Geometry check sheet. Reference: the model listing, model coordinates, mm. Face numbers are marked on the shaded views. A direction names the side the tool comes from. Give positions to 0.01 mm unless a question says otherwise; leave off trailing zeros. Loops run counter-clockwise (first coordinate to the right, second up) from the corner with the lowest first, then second, coordinate; pieces in that order, holes last.
1. Cross-section at C-C, the plane z = 0.8. Record the cut outline in (x, y).
2. Go/stop test with a flat-tipped pin: pin 1 Ø1 at (x, y) = (2.5, 5) entering from +Z. Record where the tip stops, or that it passes through.
3. Material ranges on L1, parallel to Y at x = -1.75, z = 1.2; L2, parallel to Y at x = -4, z = 4.7; L3, parallel to X at y = 0.5, z = 3.1, recorded low to high.
4. Cross-section at A-A, the plane y = 0.25. Record the cut outline in (x, z).
5. Cross-section at B-B, the plane x = -4. Record the cut outline in (y, z).
6. Cross-section at D-D, the plane x = 0.25. Record the cut outline in (y, z), plus the area to 3 significant figures.
7. Tool access check on the marked faces 1, 2 and 3. Record the directions out of +Z, -Z, +X, -X, +Y, -Y that give a thin tool (end or side, any length) a straight path to the whole face; none if there is none.
8. Release check for a two-part mould opening along Y. For the marked faces 4, 5, 6 and 7 record: +Y half, -Y half, draft (parallel to the pull), parting line (faces both ways), or undercut.
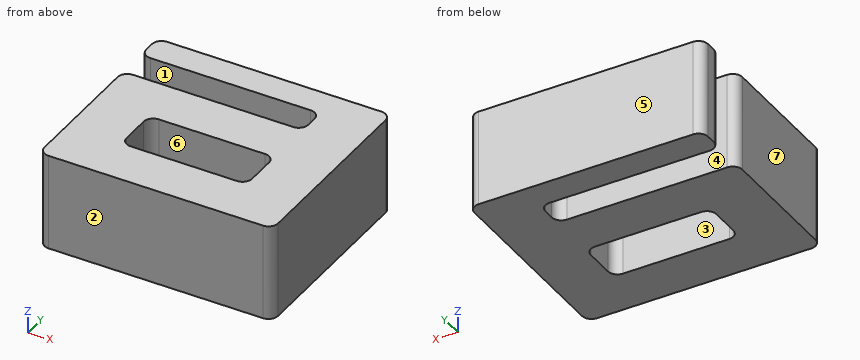
from build123d import *

# Parameters (mm, degrees)
SKETCH1_W           = 6.5
SKETCH1_H           = 2.5
BOSS_EXTRUDE1_DEPTH = 5
FILLET1_R           = 0.5


with BuildPart() as part:
    # Sketch1 → Boss-Extrude1 (new body)
    with BuildSketch(Plane.XY):
        Polygon((-6.05, -3.75), (6.05, -3.75), (6.05, 6.8), (-6.05, 6.8), (-6.05, 5.3), (3.25, 5.3), (3.25, 3.75), (-6.05, 3.75), align=None)
        Rectangle(SKETCH1_W, SKETCH1_H, mode=Mode.SUBTRACT)
    extrude(amount=BOSS_EXTRUDE1_DEPTH)

    # Fillet1
    fillet1_edges = [part.edges().sort_by_distance(p)[0] for p in [
        (-6.05, 3.75, 2.5),
        (3.25, 3.75, 2.5),
        (3.25, 5.3, 2.5),
        (-6.05, 5.3, 2.5),
        (-6.05, 6.8, 2.5),
        (6.05, 6.8, 2.5),
        (6.05, -3.75, 2.5),
        (-6.05, -3.75, 2.5),
        (-3.25, 1.25, 2.5),
        (-3.25, -1.25, 2.5),
        (3.25, -1.25, 2.5),
        (3.25, 1.25, 2.5),
    ]]
    fillet(fillet1_edges, radius=FILLET1_R)


solid = part.part
Result:
1. outline: (-6.05, -3.25) arc R0.5 ccw to (-5.55, -3.75) - (5.55, -3.75) arc R0.5 ccw to (6.05, -3.25) - (6.05, 6.3) arc R0.5 ccw to (5.55, 6.8) - (-5.55, 6.8) arc R0.5 ccw to (-6.05, 6.3) - (-6.05, 5.8) arc R0.5 ccw to (-5.55, 5.3) - (2.75, 5.3) arc R0.5 cw to (3.25, 4.8) - (3.25, 4.25) arc R0.5 cw to (2.75, 3.75) - (-5.55, 3.75) arc R0.5 ccw to (-6.05, 3.25) - close; hole (-3.25, -0.75) arc R0.5 ccw to (-2.75, -1.25) - (2.75, -1.25) arc R0.5 ccw to (3.25, -0.75) - (3.25, 0.75) arc R0.5 ccw to (2.75, 1.25) - (-2.75, 1.25) arc R0.5 ccw to (-3.25, 0.75) - close
2. pin 1: stops at z = 5
3. L1: y = -3.75 to -1.25, 1.25 to 3.75, 5.3 to 6.8
3. L2: y = -3.75 to 3.75, 5.3 to 6.8
3. L3: x = -6.05 to -3.25, 3.25 to 6.05
4. outline: (-6.05, 0) - (-3.25, 0) - (-3.25, 5) - (-6.05, 5) - close; (3.25, 0) - (6.05, 0) - (6.05, 5) - (3.25, 5) - close
5. outline: (-3.75, 0) - (3.75, 0) - (3.75, 5) - (-3.75, 5) - close; (5.3, 0) - (6.8, 0) - (6.8, 5) - (5.3, 5) - close
6. outline: (-3.75, 0) - (-1.25, 0) - (-1.25, 5) - (-3.75, 5) - close; (1.25, 0) - (3.75, 0) - (3.75, 5) - (1.25, 5) - close; (5.3, 0) - (6.8, 0) - (6.8, 5) - (5.3, 5) - close
6. area: 32.5 mm2
7. face 1: +Z, -Z, -X
7. face 2: +Z, -Z, +X, -X, -Y
7. face 3: +Z, -Z
8. face 4: undercut
8. face 5: +Y half
8. face 6: undercut
8. face 7: draft
